Source: three-view drawing plus pictorial views. Frame: mm from the lowest corner of the part. A direction names the side the tool comes from. Round coordinates to 2 decimals unless told otherwise and drop trailing zeros. Put each result on its own line as item: value. Start each with the question number.
1. Set-up query: the marked faces 1, 2, 3 and 4. Return all of +Z, -Z, +X, -X, +Y, -Y with unobstructed straight access to the full face (end or side cutting, diameter ignored); none if empty.
2. Contact query for flat-ended pins moving along their axis: pin 1 (11 mm diameter, centred on x = 17.46, z = 17.46, fed in from +Y); pin 2 (8.5 mm diameter, centred on x = 20, z = 9, fed in from -Y); pin 3 (2 mm diameter, centred on x = 51.5, y = 22.5, fed in from +Z). Output: stop coordinate, or through.
3. Material intervals for L1, parallel to Z at x = 37.5, y = 17.5; L2, parallel to Y at x = 19.5, z = 5.75; L3, parallel to X at y = 15.5, z = 5.5 (1 decimal), sorted ascending.
4. Draft query along Y for the marked faces 5, 6 and 7. Return one class per face: pulls with the +Y half, pulls with the -Y half, needs draft (parallel to the pull), parting line crosses it, or undercut.
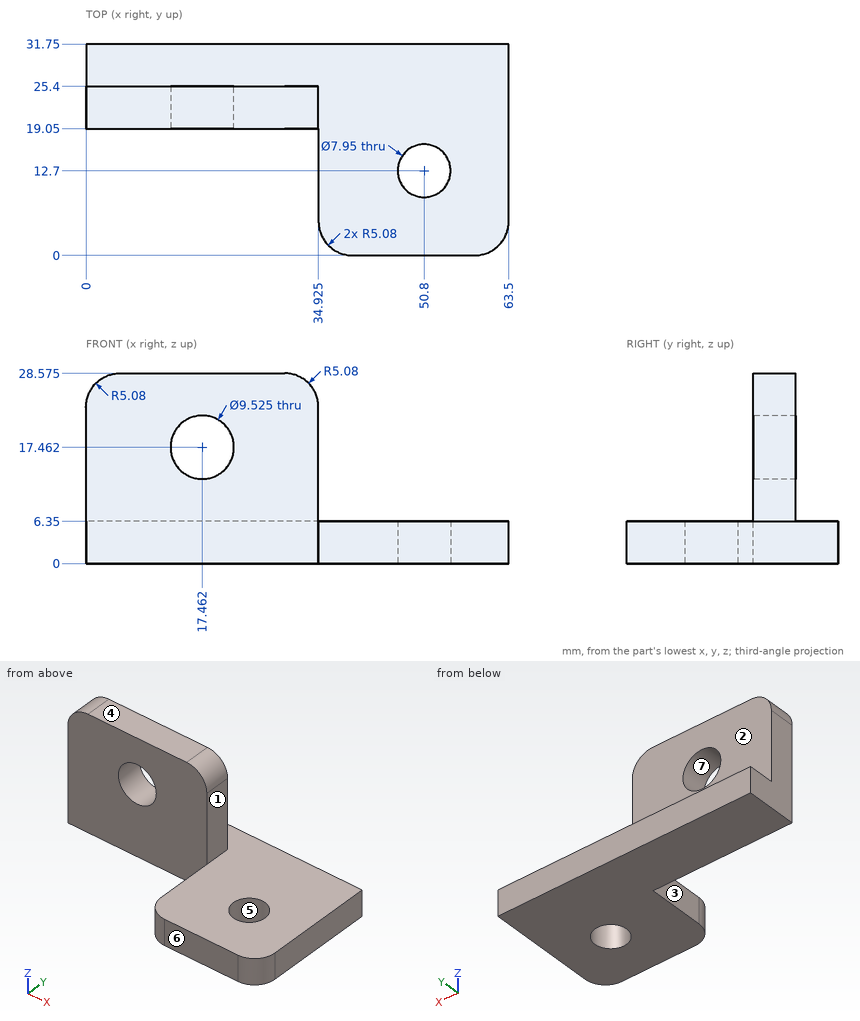
Solution:
1. face 1: +Z, +X, +Y, -Y
1. face 2: +Z, +X, -X, +Y
1. face 3: +Z, -Z, -X, -Y
1. face 4: +Z, +X, -X, +Y, -Y
2. pin 1: stops at y = 25.4
2. pin 2: stops at y = 19.05
2. pin 3: stops at z = 6.35
3. L1: z = 0 to 6.35
3. L2: y = 19.05 to 31.75
3. L3: x = 34.9 to 48, 53.6 to 63.5
4. face 5: undercut
4. face 6: pulls with the -Y half
4. face 7: needs draft
